from build123d import *

# Parameters (mm, degrees)
SKETCH1_R           = 1.5875
BOSS_EXTRUDE2_DEPTH = 4.064
SKETCH3_W           = 21.59
SKETCH3_H           = 2.032
CUT_EXTRUDE1_DEPTH  = 140.966661307
SKETCH1_7_W         = 4.388124697
SKETCH1_7_H         = 16.51
BOSS_EXTRUDE3_DEPTH = 38.1
FILLET1_R           = 5.08
FILLET2_R           = 5.08
FILLET3_R           = 5.08


with BuildPart() as part:
    # Sketch1 → Boss-Extrude2 (new body)
    with BuildSketch(Plane(origin=(0, 0, 0), x_dir=(1, 0, 0), z_dir=(0, 1, 0))):
        Polygon((2.850875303, -22.86), (60.369724697, -22.86), (60.369724697, -14.605), (89.706724697, 14.732), (89.706724697, 23.039223833), (55.9816, 29.7307), (53.8353, 31.877), (53.8353, 59.817), (55.9816, 61.9633), (89.706724697, 68.150498918), (89.706724697, 76.962), (60.369724697, 106.299), (60.369724697, 114.554), (31.6103, 114.554), (2.850875303, 114.554), (2.850875303, 106.299), (-26.486124697, 76.962), (-26.486124697, 68.150498918), (7.239, 61.9633), (9.3853, 59.817), (9.3853, 31.877), (7.239, 29.7307), (-26.486124697, 23.039223833), (-26.486124697, 14.732), (2.850875303, -14.605), align=None)
        with Locations(Location((0, 0, 0), (0, 0, 270))):
            Circle(SKETCH1_R, mode=Mode.SUBTRACT)
        with Locations(Location((-14.4272, 14.732, 0), (0, 0, 270))):
            Circle(SKETCH1_R, mode=Mode.SUBTRACT)
        Polygon((37.94125, 31.877), (55.9816, 11.69035), (37.94125, -6.35), (25.27935, -6.35), (7.239, 11.69035), (25.27935, 31.877), align=None, mode=Mode.SUBTRACT)
        with Locations(Location((63.2206, 0, 0), (0, 0, 270))):
            Circle(SKETCH1_R, mode=Mode.SUBTRACT)
        with Locations(Location((77.6478, 14.732, 0), (0, 0, 270))):
            Circle(SKETCH1_R, mode=Mode.SUBTRACT)
        with Locations(Location((-14.4272, 76.962, 0), (0, 0, 270))):
            Circle(SKETCH1_R, mode=Mode.SUBTRACT)
        with Locations(Location((0, 91.694, 0), (0, 0, 270))):
            Circle(SKETCH1_R, mode=Mode.SUBTRACT)
        Polygon((25.27935, 98.044), (37.94125, 98.044), (55.9816, 80.00365), (37.94125, 59.817), (25.27935, 59.817), (7.239, 80.00365), align=None, mode=Mode.SUBTRACT)
        with Locations(Location((77.6478, 76.962, 0), (0, 0, 270))):
            Circle(SKETCH1_R, mode=Mode.SUBTRACT)
        with Locations(Location((63.2206, 91.694, 0), (0, 0, 270))):
            Circle(SKETCH1_R, mode=Mode.SUBTRACT)
    extrude(amount=BOSS_EXTRUDE2_DEPTH)

    # Sketch3 → Cut-Extrude1 (cut, through all)
    with BuildSketch(Plane.ZY.offset(-9.3853)):
        with Locations((-45.847, 2.032)):
            Rectangle(SKETCH3_W, SKETCH3_H)
    extrude(amount=-CUT_EXTRUDE1_DEPTH, mode=Mode.SUBTRACT)

    # Sketch1_7 → Boss-Extrude3 (add)
    with BuildSketch(Plane(origin=(0, 0, 0), x_dir=(1, 0, 0), z_dir=(0, 1, 0))):
        with Locations((5.044937652, 106.299)):
            Rectangle(SKETCH1_7_W, SKETCH1_7_H)
        with Locations((58.175662348, 106.299)):
            Rectangle(SKETCH1_7_W, SKETCH1_7_H)
        with Locations((58.175662348, -14.605)):
            Rectangle(SKETCH1_7_W, SKETCH1_7_H)
        with Locations((5.044937652, -14.605)):
            Rectangle(SKETCH1_7_W, SKETCH1_7_H)
    extrude(amount=BOSS_EXTRUDE3_DEPTH)

    # Fillet1
    fillet1_edges = [part.edges().sort_by_distance(p)[0] for p in [
        (-26.486124697, 2.032, -76.962),
    ]]
    fillet(fillet1_edges, radius=FILLET1_R)

    # Fillet2
    fillet2_edges = [part.edges().sort_by_distance(p)[0] for p in [
        (-26.486124697, 2.032, -68.150498918),
    ]]
    fillet(fillet2_edges, radius=FILLET2_R)

    # Fillet3
    fillet3_edges = [part.edges().sort_by_distance(p)[0] for p in [
        (-26.486124697, 2.032, -14.732),
        (-26.486124697, 2.032, -23.039223833),
        (89.706724697, 2.032, -76.962),
        (89.706724697, 2.032, -68.150498918),
        (89.706724697, 2.032, -23.039223833),
        (89.706724697, 2.032, -14.732),
    ]]
    fillet(fillet3_edges, radius=FILLET3_R)


solid = part.part
Input: part model. Units: mm. Frame: model coordinates. A direction names the side the tool comes from. Give positions to 0.01 mm unless a question says otherwise; leave off trailing zeros. Order: outer loops, then holes, each group sorted by start corner. A loop starts at its lowest first (then second) coordinate and runs counter-clockwise, first axis right, second up. Notation, with made-up numbers: (47, -20.5) -> (106, -20.5) arc R17 ccw to (106, -16.5) -> close; hole circle Ø6 at (40.25, 83). An arc over 180 degrees is marked (long way). Use one line per item in the form item = value.
1) Mould query, pull axis Z, two halves, no side actions, for faces 6 (the flat face through (5, 38.1, 14)), 7 (the cylindrical face through (89.31, 2.06, -76.83)), 8 (the cylindrical face through (-25.3, 2.06, -22.13)). Classes: pulls with the +Z half, pulls with the -Z half, needs draft (parallel to the pull), parting line crosses it, or undercut.
Response values:
face_6 = needs draft
face_7 = pulls with the -Z half
face_8 = undercut
2) First-contact query: pin 1 Ø13 at (y, z) = (19.5, -107.5) entering from +X; pin 2 Ø1.2 at (y, z) = (2.5, -46) entering from +X; pin 3 Ø8.5 at (y, z) = (15.5, -108) entering from -X; pin 4 Ø1.9 at (x, z) = (0, -91.694) entering from +Y. Flat tips, straight axial feed; report the tip coordinate or a pass-through.
Response values:
pin_1 = 60.37
pin_2 = 53.84
pin_3 = 2.85
pin_4 = through
3) Section A-A, the plane y = 24.5. Return loops of the section in (x, z).
Response values:
outline = (2.85, -114.55) -> (7.24, -114.55) -> (7.24, -98.04) -> (2.85, -98.04) -> close; (2.85, 6.35) -> (7.24, 6.35) -> (7.24, 22.86) -> (2.85, 22.86) -> close; (55.98, -114.55) -> (60.37, -114.55) -> (60.37, -98.04) -> (55.98, -98.04) -> close; (55.98, 6.35) -> (60.37, 6.35) -> (60.37, 22.86) -> (55.98, 22.86) -> close
4) Section B-B, the plane z = 0. Return loops of the section in (x, y).
Response values:
outline = (-11.75, 0) -> (-1.59, 0) -> (-1.59, 4.06) -> (-11.75, 4.06) -> close; (1.59, 0) -> (18.93, 0) -> (18.93, 4.06) -> (1.59, 4.06) -> close; (44.29, 0) -> (61.63, 0) -> (61.63, 4.06) -> (44.29, 4.06) -> close; (64.81, 0) -> (74.97, 0) -> (74.97, 4.06) -> (64.81, 4.06) -> close
5) Line query: probe 1 along X at (y, z) = (14, 7); probe 2 along Z at (x, y) = (3, 4.5); probe 3 along Y at (x, z) = (47, -1). Output: solid intervals per line, ascending.
Response values:
probe_1 = 2.85 to 7.24, 55.98 to 60.37
probe_2 = -114.55 to -98.04, 6.35 to 22.86
probe_3 = 0 to 4.06
6) Reachability of faces 1 (the cylindrical face through (-26.11, 2.06, -14.92)), 2 (the flat face through (5, 21, 6.35)), 3 (the flat face through (47.088, 2.004, -70.052)), 4 (the flat face through (-7.37, 2.004, -26.832)), 5 (the cylindrical face through (88.52, 2.06, -22.13)) from +Z, -Z, +X, -X, +Y, -Y: full face, straight path, thin tool, end or side. Return the list, or none.
Response values:
face_1 = +Z, -X, +Y, -Y
face_2 = +X, -X, +Y
face_3 = +Y, -Y
face_4 = -X, +Y, -Y
face_5 = +X, +Y, -Y
7) Section C-C, the plane x = -19. Return loops of the section in (y, z).
Response values:
outline = (0, -84.45) -> (4.06, -84.45) -> (4.06, -66.78) -> (0, -66.78) -> close; (0, -24.52) -> (4.06, -24.52) -> (4.06, -7.25) -> (0, -7.25) -> close
